from build123d import *

# Parameters (mm, degrees)
BOSS_EXTRUDE1_DEPTH = 6.35


with BuildPart() as part:
    # Sketch2 → Boss-Extrude1 (new body)
    with BuildSketch(Plane.XY):
        with BuildLine():
            Line((8821.223823253, 3058.445977911), (8821.223823253, 3008.779305873))
            Line((8821.223823253, 3008.779305873), (8814.238823253, 3008.779305873))
            ThreePointArc((8814.238823253, 3008.779305873), (8811.993759223, 3007.849369904), (8811.063823253, 3005.604305873))
            Line((8811.063823253, 3005.604305873), (8811.063823253, 2996.079305873))
            ThreePointArc((8811.063823253, 2996.079305873), (8811.993759223, 2993.834241843), (8814.238823253, 2992.904305873))
            Line((8814.238823253, 2992.904305873), (8821.223823253, 2992.904305873))
            Line((8821.223823253, 2992.904305873), (8821.223823253, 2984.700105873))
            ThreePointArc((8821.223823253, 2984.700105873), (8819.021734877, 2979.38379425), (8813.705423253, 2977.181705873))
            Line((8813.705423253, 2977.181705873), (8813.705423253, 2980.585305873))
            Line((8813.705423253, 2980.585305873), (8801.005423253, 2980.585305873))
            Line((8801.005423253, 2980.585305873), (8801.005423253, 2977.181705873))
            Line((8801.005423253, 2977.181705873), (8760.416223253, 2977.181705873))
            Line((8760.416223253, 2977.181705873), (8760.416223253, 2980.585305873))
            Line((8760.416223253, 2980.585305873), (8747.716223253, 2980.585305873))
            Line((8747.716223253, 2980.585305873), (8747.716223253, 2977.181705873))
            ThreePointArc((8747.716223253, 2977.181705873), (8742.399911629, 2979.38379425), (8740.197823253, 2984.700105873))
            Line((8740.197823253, 2984.700105873), (8740.197823253, 2992.904305873))
            Line((8740.197823253, 2992.904305873), (8747.182823253, 2992.904305873))
            ThreePointArc((8747.182823253, 2992.904305873), (8749.427887283, 2993.834241843), (8750.357823253, 2996.079305873))
            Line((8750.357823253, 2996.079305873), (8750.357823253, 3005.604305873))
            ThreePointArc((8750.357823253, 3005.604305873), (8749.427887283, 3007.849369904), (8747.182823253, 3008.779305873))
            Line((8747.182823253, 3008.779305873), (8740.197823253, 3008.779305873))
            Line((8740.197823253, 3008.779305873), (8740.197823253, 3058.445977911))
            Line((8740.197823253, 3058.445977911), (8821.223823253, 3058.445977911))
        make_face()
        with BuildLine():
            Line((8809.285823253, 3037.151105873), (8809.285823253, 3032.985505873))
            Line((8809.285823253, 3032.985505873), (8782.631506696, 3032.985505873))
            ThreePointArc((8782.631506696, 3032.985505873), (8782.606186279, 3032.962114966), (8782.6275011, 3032.935023704))
            ThreePointArc((8782.6275011, 3032.935023704), (8780.710823253, 3008.779305873), (8778.794145406, 3032.935023704))
            ThreePointArc((8778.794145406, 3032.935023704), (8778.81546023, 3032.962114966), (8778.79013981, 3032.985505873))
            Line((8778.79013981, 3032.985505873), (8752.135823253, 3032.985505873))
            Line((8752.135823253, 3032.985505873), (8752.135823253, 3037.151105873))
            Line((8752.135823253, 3037.151105873), (8809.285823253, 3037.151105873))
        make_face(mode=Mode.SUBTRACT)
    extrude(amount=BOSS_EXTRUDE1_DEPTH)


solid = part.part
Verification items for the finished model (mm, model axes). A direction names the side the tool comes from. Coordinates: 2 decimals unless noted, no trailing zeros. Order: outer loops, then holes, each group sorted by start corner. A loop starts at its lowest first (then second) coordinate and runs counter-clockwise, first axis right, second up. Notation, with made-up numbers: (69, -15.5) -> (87, -15.5) arc R26 cw to (87, 15.5) -> close; hole circle Ø4 at (46, 67). An arc over 180 degrees is marked (long way). Put each result on its own line as item: value. Start each with the question number.
1. Mould release check, pull along X, two halves, no side actions. Record for faces 5 (the flat face through (8780, 3037.151, 3)), 6 (the flat face through (8750.358, 3001, 3)), 7 (the flat face through (8781, 2977.182, 3)): released by +X, released by -X, zero draft, split by the parting line, or undercut.
2. Cross-section at C-C, the plane x = 8785. Record the boundary of the cut face in (y, z).
3. Access from +Z, -Z, +X, -X, +Y, -Y to the whole of each face (thin tool, end or side, straight path). Record for faces 1 (the flat face through (8809.286, 3035, 3)), 2 (the flat face through (8818, 2992.904, 3)), 3 (the flat face through (8747.716, 2979, 3)), 4 (the flat face through (8744, 3008.779, 3)).
4. Material ranges on L1, parallel to Y at x = 8806.5, z = 3.75; L2, parallel to Y at x = 8785, z = 2.25; L3, parallel to X at y = 2997, z = 4.25, recorded low to high. Write a range as [from, to].
5. Cross-section at A-A, the plane x = 8806.5. Record the boundary of the cut face in (y, z).
6. Cross-section at B-B, the plane y = 3034.5. Record the boundary of the cut face in (x, z), then the cut area to 3 significant figures.
7. Go/stop test with flat-tipped pins: pin 1 Ø3 at (y, z) = (3003, 2.5) entering from +X; pin 2 Ø1.9 at (x, z) = (8817, 4) entering from -Y; pin 3 Ø2.5 at (y, z) = (2979.5, 2.5) entering from -X. Record where each tip stops, or that it passes through.
Computed:
1. face 5: undercut
1. face 6: released by -X
1. face 7: zero draft
2. outline: (2977.18, 0) -> (3009.56, 0) -> (3009.56, 6.35) -> (2977.18, 6.35) -> close; (3032.31, 0) -> (3032.99, 0) -> (3032.99, 6.35) -> (3032.31, 6.35) -> close; (3037.15, 0) -> (3058.45, 0) -> (3058.45, 6.35) -> (3037.15, 6.35) -> close
3. face 1: +Z, -Z
3. face 2: +Z, -Z, +X
3. face 3: +Z, -Z, -Y
3. face 4: +Z, -Z, -X
4. L1: [2980.59, 3032.99], [3037.15, 3058.45]
4. L2: [2977.18, 3009.56], [3032.31, 3032.99], [3037.15, 3058.45]
4. L3: [8750.36, 8811.06]
5. outline: (2980.59, 0) -> (3032.99, 0) -> (3032.99, 6.35) -> (2980.59, 6.35) -> close; (3037.15, 0) -> (3058.45, 0) -> (3058.45, 6.35) -> (3037.15, 6.35) -> close
6. outline: (8740.2, 0) -> (8752.14, 0) -> (8752.14, 6.35) -> (8740.2, 6.35) -> close; (8809.29, 0) -> (8821.22, 0) -> (8821.22, 6.35) -> (8809.29, 6.35) -> close
6. area: 152 mm2
7. pin 1: x = 8811.06
7. pin 2: y = 2977.56
7. pin 3: x = 8741.32
